Can you work these out from the drawing? Everything is in mm from the part's minimum corner. Give positions to 0.01 mm unless a question says otherwise; leave off trailing zeros. Write each loop counter-clockwise with the first axis right and the second up, starting at its lowest first coordinate (ties: lowest second). Pieces come first, ordered by that corner, then holes. Notation, with made-up numbers: (52, 11) - (89, 11) arc R8 cw to (89, 25) - close; hole circle Ø6 at (78.5, 62.5). An arc over 180 degrees is marked (long way). Use a Markdown table: item, result.
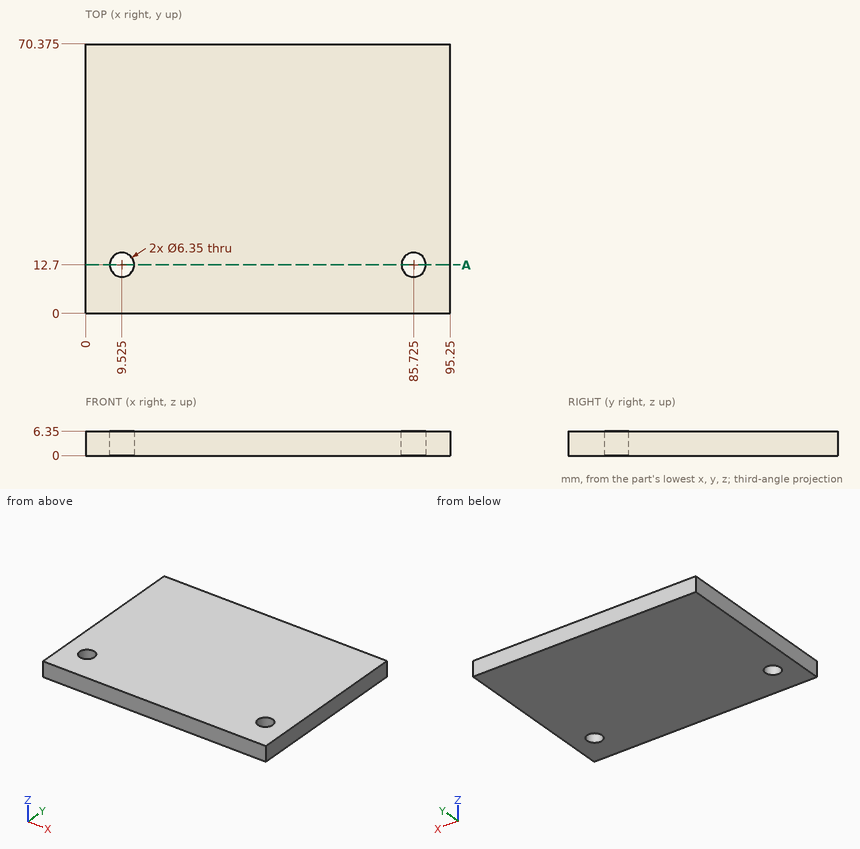
Item 1: I need wall thicknesses on line 1 along X through (y, z) = (12.5, 2.75); line 2 along Y through (x, z) = (9.5, 5) (1 decimal); line 3 along Y through (x, z) = (7.5, 2.5) (1 decimal). Which ranges of each line are inside material? Lowest first, please. Write a range as [from, to].
Values:
| item | result |
|---|---|
| line 1 | x = [0, 6.36], [12.69, 82.56], [88.89, 95.25] |
| line 2 | y = [0, 9.5], [15.9, 70.4] |
| line 3 | y = [0, 10.3], [15.1, 70.4] |
Item 2: If we section it at A-A, the plane y = 12.7: Write out the boundary of the cut face in (x, z), plus the area to 3 significant figures.
Values:
| item | result |
|---|---|
| outline | (0, 0) - (6.35, 0) - (6.35, 6.35) - (0, 6.35) - close; (12.7, 0) - (82.55, 0) - (82.55, 6.35) - (12.7, 6.35) - close; (88.9, 0) - (95.25, 0) - (95.25, 6.35) - (88.9, 6.35) - close |
| area | 524 mm2 |
Item 3: Will this pin go through, and if not, where does the flat tip stop? pin 1 Ø4 at (x, y) = (85.725, 12.7) entering from +Z.
Values:
| item | result |
|---|---|
| pin 1 | passes through |
